Study the drawing (mm; zero at the part's minimum x, y, z) and answer. Give positions to 0.01 mm unless a question says otherwise; leave off trailing zeros. Loops run counter-clockwise (first coordinate to the right, second up) from the corner with the lowest first, then second, coordinate; pieces in that order, holes last. Notation, with made-up numbers: (78, 14) - (107, 14) arc R30 ccw to (107, 42) - close; hole circle Ø9 at (28.5, 17.5). An arc over 180 degrees is marked (long way). Write item = value, one per line. Start each with the question number.
1) The part is cut by section C-C on z = 9. Write down the section's boundary in (x, y) (1 decimal).
2) The part is cut by section A-A on z = 15. Write down the section's boundary in (x, y) (1 decimal), plus the area to 3 significant figures.
3) Flat-ended cylindrical pins translate along their axes: P1, Ø3.5, axis at y = 37, z = 8.5, coming from the +X side; P2, Ø16, axis at x = 22, z = 11.5, coming from the -Y side (1 decimal); P3, Ø10.5, axis at x = 40.5, y = 28.5, coming from the -Z side (1 decimal). Find the tip coordinate at first contact, or state that the pin passes through.
4) Consider probe 1 along Y at (x, z) = (17.5, 20.5) (1 decimal); probe 2 along X at (y, z) = (36, 7); probe 3 along Z at (x, y) = (13, 3). Determine where each line is inside the solid, lowest interval first.
5) The mould has two halves that part along Z. Classify the marked faces 1, 2 and 3: +Z half, -Z half, draft (parallel to the pull), parting line (faces both ways), or undercut.
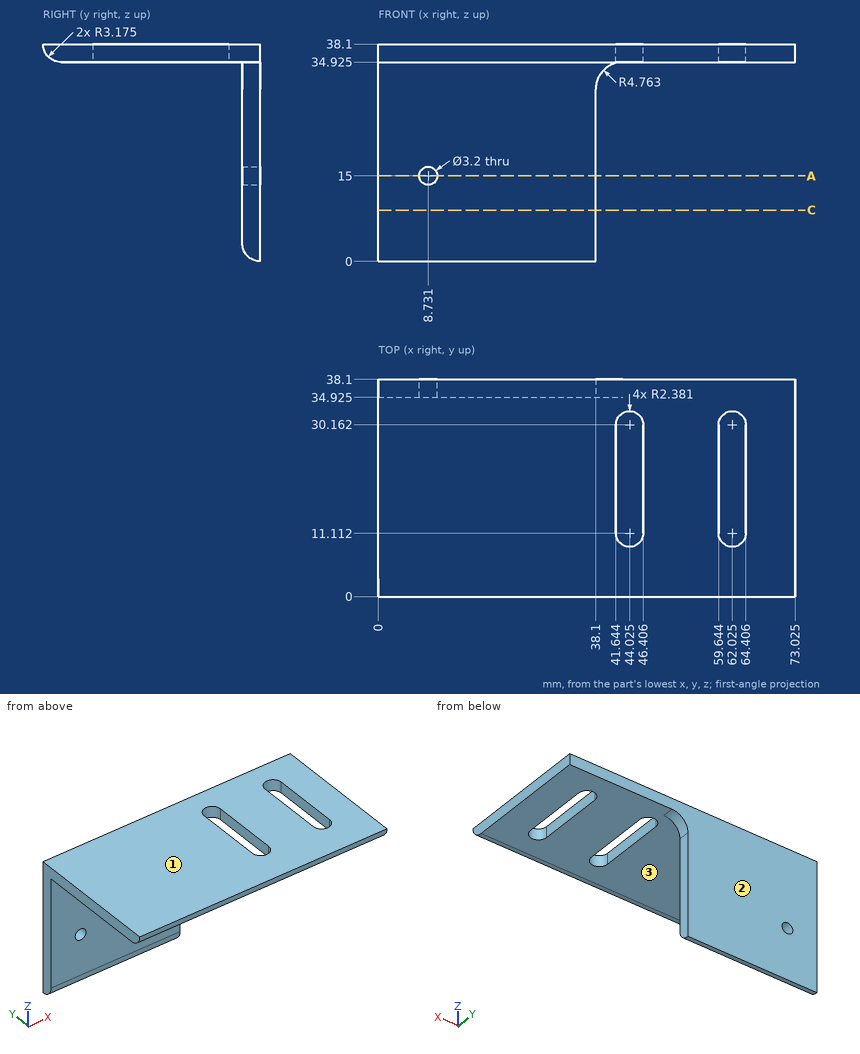
Answer below:
q1.outline = (0, 34.9) - (38.1, 34.9) - (38.1, 38.1) - (0, 38.1) - close
q2.outline = (0, 34.9) - (7.1, 34.9) - (7.1, 38.1) - (0, 38.1) - close; (10.3, 34.9) - (38.1, 34.9) - (38.1, 38.1) - (10.3, 38.1) - close
q2.area = 111 mm2
q3.P1 = 38.1
q3.P2 = 34.9
q3.P3 = 34.9
q4.probe_1 = 34.9 to 38.1
q4.probe_2 = 0 to 38.1
q4.probe_3 = 34.93 to 38.1
q5.face_1 = +Z half
q5.face_2 = draft
q5.face_3 = -Z half
